```python
from build123d import *

# Parameters (mm, degrees)
PAD001_DEPTH  = 2
FILLET004_R   = 7
FILLET013_R   = 2
FILLET005_R   = 1
FILLET006_R   = 1.2
SKETCH014_R   = 1.7
HOLE003_DEPTH = 25


with BuildPart() as part:
    # Sketch001 → Pad001 (new body)
    with BuildSketch(Plane.XY):
        Polygon((-152.075, 56.825), (152.075, 56.825), (152.075, -40.775), (108.5, -52.5375), (94.2125, -66.825), (-113.2625, -66.825), (-127.55, -52.5375), (-152.075, -40.775), align=None)
        Polygon((143.075, 47.825), (-143.075, 47.825), (-143.075, -28.775), (-119.2625, -28.775), (-119.2625, -47.825), (100.2125, -47.825), (100.2125, -28.775), (143.075, -28.775), align=None, mode=Mode.SUBTRACT)
    extrude(amount=-PAD001_DEPTH)

    # Fillet004
    fillet004_edges = [part.edges().sort_by_distance(p)[0] for p in [
        (152.075, 56.825, -1),
        (108.5, -52.5375, -1),
        (94.2125, -66.825, -1),
        (-113.2625, -66.825, -1),
        (-127.55, -52.5375, -1),
        (-152.075, 56.825, -1),
    ]]
    fillet(fillet004_edges, radius=FILLET004_R)

    # Fillet013
    fillet013_edges = [part.edges().sort_by_distance(p)[0] for p in [
        (-152.075, -40.775, -1),
        (152.075, -40.775, -1),
    ]]
    fillet(fillet013_edges, radius=FILLET013_R)

    # Fillet005
    fillet005_edges = [part.edges().sort_by_distance(p)[0] for p in [
        (143.075, 47.825, -1),
        (143.075, -28.775, -1),
        (100.2125, -47.825, -1),
        (-143.075, -28.775, -1),
        (-119.2625, -47.825, -1),
        (-143.075, 47.825, -1),
    ]]
    fillet(fillet005_edges, radius=FILLET005_R)

    # Fillet006
    fillet006_edges = [part.edges().sort_by_distance(p)[0] for p in [
        (-119.2625, -28.775, -1),
        (100.2125, -28.775, -1),
    ]]
    fillet(fillet006_edges, radius=FILLET006_R)

    # Sketch014 (on Face1 of Fillet006) → Hole003 (cut)
    with BuildSketch(Plane.XY):
        with Locations((147.575, 52.325)):
            Circle(SKETCH014_R)
        with Locations((147.575, -19.05)):
            Circle(SKETCH014_R)
        with Locations((57.15, -52.325)):
            Circle(SKETCH014_R)
        with Locations((-57.15, -52.325)):
            Circle(SKETCH014_R)
        with Locations((-147.575, -19.05)):
            Circle(SKETCH014_R)
        with Locations((-147.575, 52.325)):
            Circle(SKETCH014_R)
        with Locations((-38.1, 52.325)):
            Circle(SKETCH014_R)
        with Locations((38.1, 52.325)):
            Circle(SKETCH014_R)
    extrude(amount=-HOLE003_DEPTH, mode=Mode.SUBTRACT)


solid = part.part
```
The model under review builds one solid part; all positions refer to its coordinate system, in mm. Give positions to 0.01 mm unless a question says otherwise; leave off trailing zeros. Write each loop counter-clockwise with the first axis right and the second up, starting at its lowest first coordinate (ties: lowest second). Pieces come first, ordered by that corner, then holes. Notation, with made-up numbers: M 59,-34 L 106,-34 A29 ccw 106,-1 Z; hole C -28.5,-25.75 d8. An arc over 180 degrees is marked long. Write each question's results on one line, items separated by ' | '. Start each with the question number.
1. We need section A-A (x = -73). Write out the cut boundary in (y, z) (3 decimals), and give its area (3 significant figures).
2. We need section B-B (y = 28). Write out the cut boundary in (x, z) (3 decimals), and give its area (3 significant figures).
3. We need section C-C (z = -1.2). Count the separate pieces of the cut face and the enclosed holes in it, and give its area (4 significant figures).
4. For probe 1 along X at (y, z) = (10, -1.55) (3 decimals); probe 2 along Y at (x, z) = (19, -1.2) (3 decimals); probe 3 along X at (y, z) = (-35.5, -1.3) (1 decimal), list the stretches that pass through material, from the lowest coordinate up. Write a range as [from, to].
Results found:
1) outline: M -66.825,-2 L -47.825,-2 L -47.825,0 L -66.825,0 Z; M 47.825,-2 L 56.825,-2 L 56.825,0 L 47.825,0 Z | area: 56.0 mm^2
2) outline: M -152.075,-2 L -143.075,-2 L -143.075,0 L -152.075,0 Z; M 143.075,-2 L 152.075,-2 L 152.075,0 L 143.075,0 Z | area: 36.0 mm^2
3) separate pieces: 1 | enclosed holes: 9 | area: 9,835 mm^2
4) probe 1: x = [-152.075, -143.075], [143.075, 152.075] | probe 2: y = [-66.825, -47.825], [47.825, 56.825] | probe 3: x = [-152.1, -119.3], [100.2, 152.1]
